Verification items for the finished model (mm, model axes). A direction names the side the tool comes from. Give positions to 0.01 mm unless a question says otherwise; leave off trailing zeros. Order: outer loops, then holes, each group sorted by start corner. A loop starts at its lowest first (then second) coordinate and runs counter-clockwise, first axis right, second up. Notation, with made-up numbers: (-25, 10.25) - (-1, 10.25) arc R32 ccw to (-1, 38.25) - close; hole circle Ø5 at (-11.5, 33). An arc over 180 degrees is marked (long way). Answer as a JSON object with one key per item and string values. Group by question number.
(1) Access from +Z, -Z, +X, -X, +Y, -Y to the whole of each face (thin tool, end or side, straight path). Record for faces 1 (the face through (8.62, -36.51, 5.07)), 2 (the face through (-8.62, -36.51, -5.07)), 3 (the face through (8.7, -36.51, -4.93)), 4 (the face through (-8.7, -36.51, 4.93)).
(2) Section check C-C (z = 2). Record the boundary of the cut face in (x, y).
(3) Thickness scan on line 1 (X direction, y = -6.5, z = -17.5); line 2 (Z direction, x = -2, y = -12); line 3 (X direction, y = -25, z = -9). Record the ranges inside material, lowest first.
(4) Section check D-D (y = -12.5). Record the boundary of the cut face in (x, z), then the cut area to 3 significant figures.
(5) Section check A-A (x = 0). Record the boundary of the cut face in (y, z), then the cut area to 3 significant figures.
(6) Section check B-B (y = -42). Record the boundary of the cut face in (x, z).
(7) Depth check by flat-ended pin: pin 1 Ø3.5 at (x, y) = (-1, -30.5) entering from +Z; pin 2 Ø1 at (y, z) = (-0.5, 13) entering from -X; pin 3 Ø3 at (y, z) = (-16, -9.5) entering from +X. Enter the tip coordinate at first touch or a pass-through.
```python
from build123d import *

# Parameters (mm, degrees)
BOSS_EXTRUDE1_DEPTH = 50.8


with BuildPart() as part:
    # Sketch2 → Revolve3 (revolve)
    with BuildSketch(Plane.XY):
        with BuildLine():
            Line((0, 12.7), (0, -25.4))
            ThreePointArc((0, -25.4), (17.960512242, -17.960512242), (25.4, 0))
            Line((25.4, 0), (25.4, 12.7))
            Line((25.4, 12.7), (0, 12.7))
        make_face()
    revolve(axis=Axis((0, -50, 0), (0, 1, 0)))

    # Sketch3 → Boss-Extrude1 (add)
    with BuildSketch(Plane(origin=(0, 0, 0), x_dir=(1, 0, 0), z_dir=(0, 1, 0))):
        Polygon((-5.773502692, -10), (5.773502692, -10), (11.547005384, 0), (5.773502692, 10), (-5.773502692, 10), (-11.547005384, 0), align=None)
    extrude(amount=-BOSS_EXTRUDE1_DEPTH)


solid = part.part
```
Solutions:
{
 "1": {"face 1": "+Z, +X, -Y", "face 2": "-Z, -X, -Y", "face 3": "-Z, +X, -Y", "face 4": "+Z, -X, -Y"},
 "2": {"outline": "(-25.32, 0) arc R25.32 ccw to (-10.39, -23.09) - (-10.39, -50.8) - (10.39, -50.8) - (10.39, -23.09) arc R25.32 ccw to (25.32, 0) - (25.32, 12.7) - (-25.32, 12.7) - close"},
 "3": {"line 1": "x = -17.22 to 17.22", "line 2": "z = -22.3 to 22.3", "line 3": "x = -6.35 to 6.35"},
 "4": {"outline": "circle Ø44.22 at (0, 0)", "area": "1,540 mm2"},
 "5": {"outline": "(-50.8, -10) - (-23.35, -10) arc R25.4 ccw to (0, -25.4) - (12.7, -25.4) - (12.7, 25.4) - (0, 25.4) arc R25.4 ccw to (-23.35, 10) - (-50.8, 10) - close", "area": "2,180 mm2"},
 "6": {"outline": "(-11.55, 0) - (-5.77, -10) - (5.77, -10) - (11.55, 0) - (5.77, 10) - (-5.77, 10) - close"},
 "7": {"pin 1": "stops at z = 10", "pin 2": "stops at x = -22.11", "pin 3": "stops at x = 18.77"}
}
